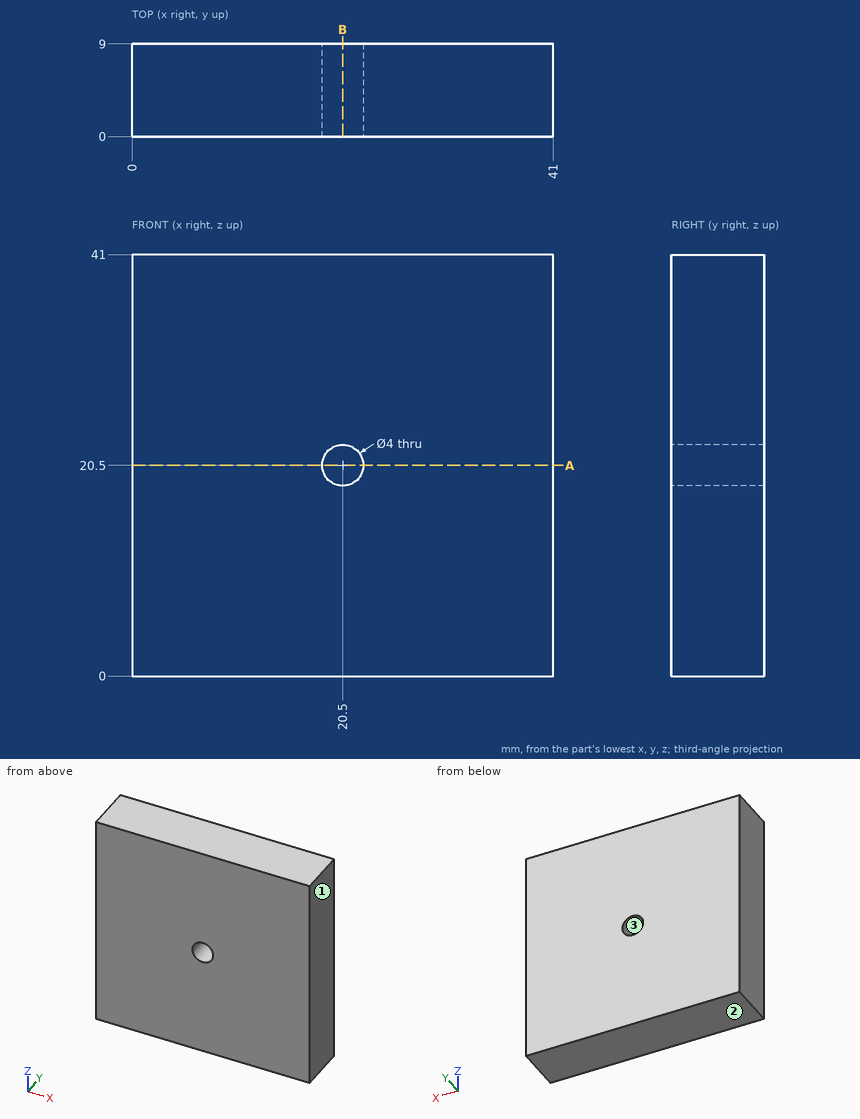
For this review, use the dimensioned drawing (mm, ordinates from the lowest corner) and the shaded views. Give positions to 0.01 mm unless a question says otherwise; leave off trailing zeros. Order: outer loops, then holes, each group sorted by start corner. A loop starts at its lowest first (then second) coordinate and runs counter-clockwise, first axis right, second up. Notation, with made-up numbers: (17, 77) -> (30, 77) arc R23 cw to (30, 108) -> close; hole circle Ø4 at (-34.75, -8.5). An arc over 180 degrees is marked (long way). Write item = value, one per line. Start each with the question number.
(1) Draft analysis for pull direction X (two halves, no side actions). For the marked faces 1, 2 and 3, state which applies: +X half, -X half, draft (parallel to the pull), parting line (faces both ways), or undercut.
(2) Take a section at A-A (z = 20.5). Write out the cut boundary in (x, y), plus the area to 3 significant figures.
(3) For L1, parallel to Z at x = 20.5, y = 4.25; L2, parallel to Z at x = 20, y = 4.5, list the stretches that pass through material, from the lowest coordinate up. Write a range as from..to.
(4) Take a section at B-B (x = 20.5). Write out the cut boundary in (y, z), plus the area to 3 significant figures.
Returned:
q1.face_1 = +X half
q1.face_2 = draft
q1.face_3 = undercut
q2.outline = (0, 0) -> (18.5, 0) -> (18.5, 9) -> (0, 9) -> close; (22.5, 0) -> (41, 0) -> (41, 9) -> (22.5, 9) -> close
q2.area = 333 mm²
q3.L1 = 0..18.5, 22.5..41
q3.L2 = 0..18.56, 22.44..41
q4.outline = (0, 0) -> (9, 0) -> (9, 18.5) -> (0, 18.5) -> close; (0, 22.5) -> (9, 22.5) -> (9, 41) -> (0, 41) -> close
q4.area = 333 mm²
